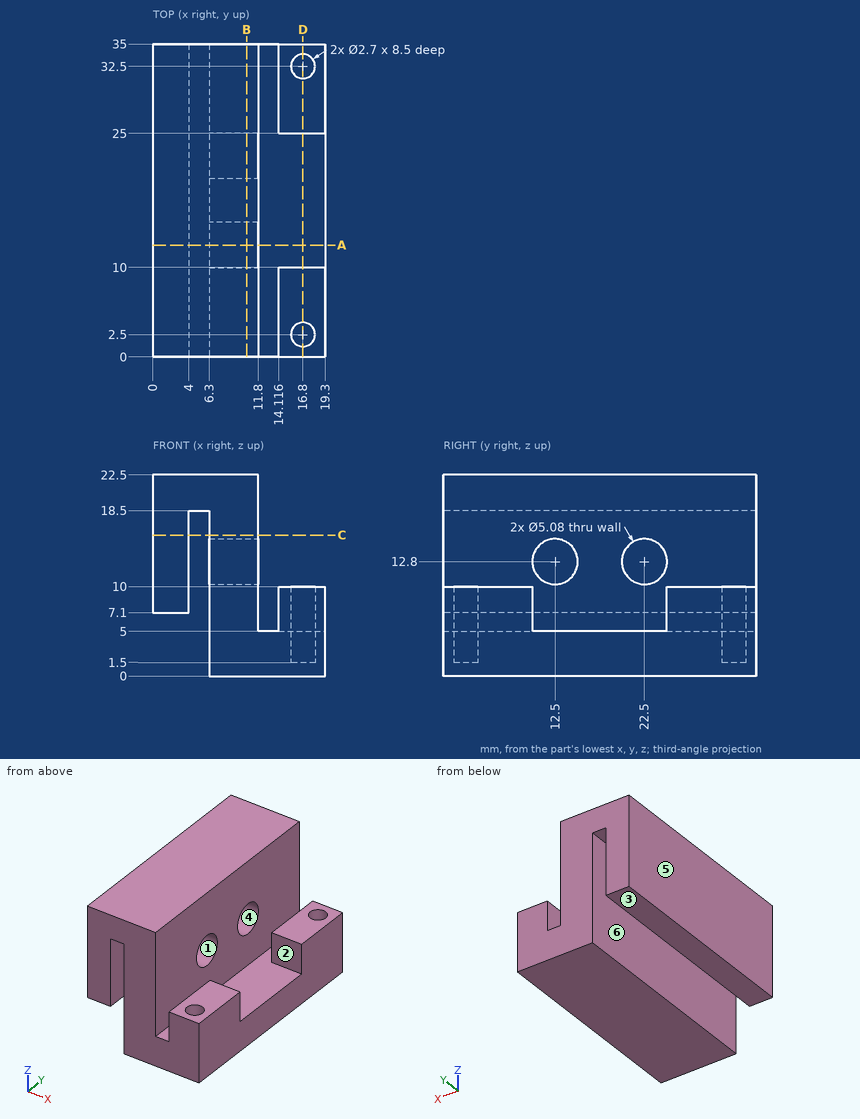
Study the drawing (mm; zero at the part's minimum x, y, z) and answer. A direction names the side the tool comes from. Coordinates: 2 decimals unless noted, no trailing zeros. Write each loop counter-clockwise with the first axis right and the second up, starting at its lowest first coordinate (ties: lowest second). Pieces come first, ordered by that corner, then holes. Notation, with made-up numbers: M 74,28 L 83,28 A27 ccw 83,52 Z; hole C 30.25,22.25 d8. An arc over 180 degrees is marked long. Write each question's results on one line, items separated by ' | '.
Item 1: The part is cut by section C-C on z = 15.75. Determine the outline of the cut face in (x, y).
Answer below:
outline: M 0,0 L 4,0 L 4,35 L 0,35 Z; M 6.3,0 L 11.8,0 L 11.8,35 L 6.3,35 Z
Item 2: Consider probe 1 along Y at (x, z) = (16.8, 6); probe 2 along X at (y, z) = (27, 10.25); probe 3 along Z at (x, y) = (9, 12.5). Determine where each line is inside the solid, lowest interval first. Write a range as [from, to].
Answer below:
probe 1: [0, 1.15], [3.85, 10], [25, 31.15], [33.85, 35] | probe 2: [0, 4], [6.3, 11.8] | probe 3: [0, 10.26], [15.34, 22.5]
Item 3: The part is cut by section B-B on x = 10.5. Determine the outline of the cut face in (y, z), and give its area (3 significant figures).
Answer below:
outline: M 0,0 L 35,0 L 35,22.5 L 0,22.5 Z; hole C 12.5,12.8 d5.08; hole C 22.5,12.8 d5.08 | area: 747 mm2
Item 4: The part is cut by section D-D on x = 16.8. Determine the outline of the cut face in (y, z).
Answer below:
outline: M 0,0 L 35,0 L 35,10 L 33.85,10 L 33.85,1.5 L 31.15,1.5 L 31.15,10 L 25,10 L 25,5 L 10,5 L 10,10 L 3.85,10 L 3.85,1.5 L 1.15,1.5 L 1.15,10 L 0,10 Z
Item 5: The part is cut by section A-A on y = 12.5. Determine the outline of the cut face in (x, z).
Answer below:
outline: M 0,7.1 L 4,7.1 L 4,18.5 L 6.3,18.5 L 6.3,15.34 L 11.8,15.34 L 11.8,22.5 L 0,22.5 Z; M 6.3,0 L 19.3,0 L 19.3,5 L 11.8,5 L 11.8,10.26 L 6.3,10.26 Z
Item 6: Given P1, Ø2.5, axis at x = 18, y = 2.5, coming from the +Z side; P2, Ø1.5, axis at x = 17, z = 7, coming from the -Y side; P3, Ø4.5, axis at x = 2, y = 17.5, coming from the -Z side; P4, Ø2, axis at x = 17, y = 17, coming from the +Z side, each flat-ended and moving along its own axis, determine where each tip first touches the part or whether it passes through.
Answer below:
P1: z = 10 | P2: y = 0 | P3: z = 7.1 | P4: z = 5
Item 7: For a pull along X with two mould halves and no side action, classify the marked faces 4, 5 and 6 as released by +X, released by -X, zero draft, split by the parting line, or undercut.
Answer below:
face 4: zero draft | face 5: released by -X | face 6: undercut
Item 8: Which of the six approach directions +Z, -Z, +X, -X, +Y, -Y give full straight-line access (tool end or side, diameter ignored) to the marked faces 1, 2 and 3?
Answer below:
face 1: +X | face 2: +Z, +X | face 3: -Z, -X, +Y, -Y
